CAD build for the part. Positions are in the model's coordinates, mm. A direction names the side the tool comes from. Coordinates: 2 decimals unless noted, no trailing zeros. Loops run counter-clockwise (first coordinate to the right, second up) from the corner with the lowest first, then second, coordinate; pieces in that order, holes last.
1) Which spindle directions (+Z, -Z, +X, -X, +Y, -Y) get a long thin tool onto all of the face, cutting with end or side? Do faces 1 (the flat face through (-6, 10, 49)), 2 (the flat face through (-8.667, -4, 49)). Say none if no direction does.
2) Wall check: line 1 along Y through (x, z) = (-7.75, 42.5); line 2 along Y through (x, z) = (3, 43.5); line 3 along X through (y, z) = (-7.5, 88.5). Give the ranges that are in metal, low to high.
3) Saw through at C-C, the plane z = 47.5. Give the number of separate pieces and of enclosed holes in the cut face, and give its area (3 significant figures).
4) Two-plate mould, pull along X, no slides. Class faces 3 (the flat face through (6, 10, 49)), 4 (the flat face through (10, -6, 49)), 5 (the flat face through (-4.996, -4.309, 49.3)): +X half, -X half, draft (parallel to the pull), parting line (faces both ways), or undercut.
5) Saw through at A-A, the plane y = 0. Write the cut outline in (x, z).
```python
from build123d import *

# Parameters (mm, degrees)
SKETCH3_R           = 1.400007
SKETCH3_R_2         = 2.266678
BOSS_EXTRUDE1_DEPTH = 100


with BuildPart() as part:
    # Sketch3 → Boss-Extrude1 (new body)
    with BuildSketch(Plane.XY):
        Polygon((8.66671, -5.5000275), (6.019640257, -5.5000275), (4.00002, -3.150816419), (4.00002, 0), (4.00002, 3.150816419), (6.019640257, 5.5000275), (8.66671, 5.5000275), (8.66671, 2.66668), (10.00005, 2.66668), (10.00005, 10.00005), (2.66668, 10.00005), (2.66668, 8.66671), (5.5000275, 8.66671), (5.5000275, 6.019640257), (3.150816419, 4.00002), (0, 4.00002), (-3.150816419, 4.00002), (-5.5000275, 6.019640257), (-5.5000275, 8.66671), (-2.66668, 8.66671), (-2.66668, 10.00005), (-10.00005, 10.00005), (-10.00005, 2.66668), (-8.66671, 2.66668), (-8.66671, 5.5000275), (-6.019640257, 5.5000275), (-4.00002, 3.150816419), (-4.00002, 0), (-4.00002, -3.150816419), (-6.019640257, -5.5000275), (-8.66671, -5.5000275), (-8.66671, -2.66668), (-10.00005, -2.66668), (-10.00005, -10.00005), (-2.66668, -10.00005), (-2.66668, -8.66671), (-5.5000275, -8.66671), (-5.5000275, -6.019640257), (-3.150816419, -4.00002), (0, -4.00002), (3.150816419, -4.00002), (5.5000275, -6.019640257), (5.5000275, -8.66671), (2.66668, -8.66671), (2.66668, -10.00005), (10.00005, -10.00005), (10.00005, -2.66668), (8.66671, -2.66668), align=None)
        with Locations((7.733372, -7.733372)):
            Circle(SKETCH3_R, mode=Mode.SUBTRACT)
        with Locations((7.733372, 7.733372)):
            Circle(SKETCH3_R, mode=Mode.SUBTRACT)
        with Locations((-7.733372, 7.733372)):
            Circle(SKETCH3_R, mode=Mode.SUBTRACT)
        Circle(SKETCH3_R_2, mode=Mode.SUBTRACT)
        with Locations((-7.733372, -7.733372)):
            Circle(SKETCH3_R, mode=Mode.SUBTRACT)
    extrude(amount=BOSS_EXTRUDE1_DEPTH)


solid = part.part
```
Data:
1. face 1: +Z, -Z, +X, -X, +Y
1. face 2: +Z, -Z
2. line 1: y = -10 to -9.13, -6.33 to -5.5, 5.5 to 6.33, 9.13 to 10
2. line 2: y = -10 to -8.67, -4 to 4, 8.67 to 10
2. line 3: x = -10 to -9.11, -6.35 to -5.5, 5.5 to 6.35, 9.11 to 10
3. separate pieces: 1
3. enclosed holes: 5
3. area: 144 mm2
4. face 3: draft
4. face 4: +X half
4. face 5: undercut
5. outline: (-4, 0) - (-2.27, 0) - (-2.27, 100) - (-4, 100) - close; (2.27, 0) - (4, 0) - (4, 100) - (2.27, 100) - close
